Check sheet for the modelled part. Datum: model origin and axes. Units: mm. A direction names the side the tool comes from. Coordinates: 2 decimals unless noted, no trailing zeros. Order: outer loops, then holes, each group sorted by start corner. A loop starts at its lowest first (then second) coordinate and runs counter-clockwise, first axis right, second up.
from build123d import *

# Parameters (mm, degrees)
EXTRUDE_1_DEPTH     = 20
EXTRUDE_2_DEPTH     = 3
EXTRUDE_3_DEPTH     = 3
CHAMFER_1_SIZE      = 10
SKETCH_4_R          = 2.1
CUT_EXTRUDE_1_DEPTH = 3
CUT_EXTRUDE_2_DEPTH = 10
FILLET_1_R          = 1
SKETCH_6_R          = 2.1
CUT_EXTRUDE_3_DEPTH = 10
SKETCH_7_R          = 3.5
CUT_EXTRUDE_4_DEPTH = 10
SKETCH_8_W          = 10
SKETCH_8_H          = 10
CUT_EXTRUDE_5_DEPTH = 7
FILLET_2_R          = 1
SKETCH_9_R          = 3.5
CUT_EXTRUDE_6_DEPTH = 1
SKETCH_10_R         = 3.5
CUT_EXTRUDE_7_DEPTH = 1


with BuildPart() as part:
    # 草图1 → 凸台-拉伸1 (new body)
    with BuildSketch(Plane(origin=(0, 0, 0), x_dir=(1, 0, 0), z_dir=(0, 1, 0))):
        Polygon((0, 20), (0, 0), (20, 0), (20, 3), (3, 3), (3, 20), align=None)
    extrude(amount=EXTRUDE_1_DEPTH)

    # 草图2 → 凸台-拉伸2 (add)
    with BuildSketch(Plane(origin=(0, 20, 0), x_dir=(1, 0, 0), z_dir=(0, 1, 0))):
        Polygon((3, 20), (20, 3), (3, 3), align=None)
    extrude(amount=-EXTRUDE_2_DEPTH)

    # 草图3 → 凸台-拉伸3 (add)
    with BuildSketch(Plane.XZ):
        Polygon((20, -3), (3, -20), (3, -3), align=None)
    extrude(amount=-EXTRUDE_3_DEPTH)

    # 倒角1
    chamfer_1_edges = [part.edges().sort_by_distance(p)[0] for p in [
        (3, 10, -3),
    ]]
    chamfer(chamfer_1_edges, length=CHAMFER_1_SIZE)

    # 草图4 → 切除-拉伸1 (cut)
    with BuildSketch(Plane(origin=(0, 0, -3), x_dir=(-1, 0, 0), z_dir=(0, 0, -1))):
        with Locations((-10, 10)):
            Circle(SKETCH_4_R)
    extrude(amount=-CUT_EXTRUDE_1_DEPTH, mode=Mode.SUBTRACT)

    # 草图5 → 切除-拉伸2 (cut)
    with BuildSketch(Plane(origin=(0, 0, -3), x_dir=(-1, 0, 0), z_dir=(0, 0, -1))):
        with BuildLine():
            Line((-10, 13.5), (-13, 13.5))
            Line((-13, 13.5), (-13, 6.5))
            Line((-13, 6.5), (-10, 6.5))
            ThreePointArc((-10, 6.5), (-6.5, 10), (-10, 13.5))
        make_face()
    extrude(amount=CUT_EXTRUDE_2_DEPTH, mode=Mode.SUBTRACT)

    # 圆角1
    fillet_1_edges = [part.edges().sort_by_distance(p)[0] for p in [
        (11.5, 20, -11.5),
        (11.5, 0, -11.5),
    ]]
    fillet(fillet_1_edges, radius=FILLET_1_R)

    # 草图6 → 切除-拉伸3 (cut)
    with BuildSketch(Plane(origin=(3, 0, 0), x_dir=(0, 0, -1), z_dir=(1, 0, 0))):
        with Locations((10, 10)):
            Circle(SKETCH_6_R)
    extrude(amount=-CUT_EXTRUDE_3_DEPTH, mode=Mode.SUBTRACT)

    # 草图7 → 切除-拉伸4 (cut)
    with BuildSketch(Plane.ZY.offset(-3)):
        with Locations((-10, 10)):
            Circle(SKETCH_7_R)
    extrude(amount=-CUT_EXTRUDE_4_DEPTH, mode=Mode.SUBTRACT)

    # 草图8 → 切除-拉伸5 (cut)
    with BuildSketch(Plane.XZ.offset(-13.5)):
        with Locations((8, -8)):
            Rectangle(SKETCH_8_W, SKETCH_8_H)
    extrude(amount=CUT_EXTRUDE_5_DEPTH, mode=Mode.SUBTRACT)

    # 圆角2
    fillet_2_edges = [part.edges().sort_by_distance(p)[0] for p in [
        (8, 3, -8),
        (8, 17, -8),
        (8, 13.5, -8),
        (8, 6.5, -8),
    ]]
    fillet(fillet_2_edges, radius=FILLET_2_R)

    # 草图9 → 切除-拉伸6 (cut)
    with BuildSketch(Plane(origin=(0, 0, -3), x_dir=(-1, 0, 0), z_dir=(0, 0, -1))):
        with Locations((-10, 10)):
            Circle(SKETCH_9_R)
    extrude(amount=-CUT_EXTRUDE_6_DEPTH, mode=Mode.SUBTRACT)

    # 草图10 → 切除-拉伸7 (cut)
    with BuildSketch(Plane(origin=(3, 0, 0), x_dir=(0, 0, -1), z_dir=(1, 0, 0))):
        with Locations((10, 10)):
            Circle(SKETCH_10_R)
    extrude(amount=-CUT_EXTRUDE_7_DEPTH, mode=Mode.SUBTRACT)


solid = part.part
(1) Tool access check on faces 5 (the flat face through (20, 10, -1)), 6 (the flat face through (6, 13.5, -6)), 7 (the flat face through (8, 8, -2)). Record the directions out of +Z, -Z, +X, -X, +Y, -Y that give a thin tool (end or side, any length) a straight path to the whole face; none if there is none.
Filled in:
face 5: +Z, -Z, +X, +Y, -Y
face 6: -Z, +X
face 7: -Z
(2) Thickness scan on probe 1 along Z at (x, y) = (2.2, 10); probe 2 along Y at (x, z) = (10, -1.2); probe 3 along Y at (x, z) = (2.65, -10). Record the ranges inside material, lowest first.
Filled in:
probe 1: z = -20 to -13.5, -6.5 to 0
probe 2: y = 0 to 7.9, 12.1 to 20
probe 3: y = 0 to 6.5, 13.5 to 20
(3) Go/stop test with flat-tipped pins: P1, Ø5.5, axis at y = 10.5, z = -11, coming from the +X side; P2, Ø5.5, axis at x = 10, y = 10, coming from the +Z side; P3, Ø9, axis at x = 10, y = 10, coming from the -Z side; P4, Ø4, axis at y = 10, z = -10, coming from the +X side. Record where each tip stops, or that it passes through.
Filled in:
P1: stops at x = 3
P2: stops at z = 0
P3: stops at z = -8.01
P4: passes through
(4) Release check for a two-part mould opening along Z. For faces 1 (the flat face through (0, 9.9, -12.4)), 2 (the flat face through (9.9, 7.6, 0)), 3 (the flat face through (16, 10, -3)), 4 (the cylindrical face through (1.01, 10.09, -7.9)) record: +Z half, -Z half, draft (parallel to the pull), parting line (faces both ways), or undercut.
Filled in:
face 1: draft
face 2: +Z half
face 3: -Z half
face 4: undercut
(5) Cross-section at A-A (y = 11). Enter the section's corners in (x, z).
Filled in:
outline: (0, -20) - (3, -20) - (3, -13.35) - (2, -13.35) - (2, -11.85) - (0, -11.85) - close; (0, -8.15) - (2, -8.15) - (2, -6.65) - (3, -6.65) - (3, -3) - (6.65, -3) - (6.65, -2) - (8.15, -2) - (8.15, 0) - (0, 0) - close; (11.85, -2) - (13.35, -2) - (13.35, -3) - (20, -3) - (20, 0) - (11.85, 0) - close
